from build123d import *

# Parameters (mm, degrees)
F3_DEPTH = 8
F4_R     = 0.4
F5_R     = 0.5


with BuildPart() as f1:
    # F0 (on Right) → F1 (revolve)
    with BuildSketch(Plane.YZ):
        Polygon((0, -60), (0, 0), (-7.95, 0), (-7.95, -10), (-5, -10), (-5, -60), align=None)
    revolve(axis=Axis((0, 0, -30), (0, 0, -1)))

    # F2 (on face) → F3 (cut)
    with BuildSketch(Plane.XY):
        Polygon((-2.341641, 3.981212), (-4.618651, -0.037314), (-2.277011, -4.018527), (2.341641, -3.981212), (4.618651, 0.037314), (2.277011, 4.018527), align=None)
    extrude(amount=-F3_DEPTH, mode=Mode.SUBTRACT)

    # F4
    f4_edges = [f1.edges().sort_by_distance(p)[0] for p in [
        (0, 7.95, 0),
        (0, 7.95, -10),
    ]]
    fillet(f4_edges, radius=F4_R)

    # F5
    f5_edges = [f1.edges().sort_by_distance(p)[0] for p in [
        (0, 5, -10),
        (0, 5, -60),
    ]]
    fillet(f5_edges, radius=F5_R)


solid = f1.part
Geometry: final body of the model. Coordinates: model frame, mm. A direction names the side the tool comes from. Coordinates: 2 decimals unless noted, no trailing zeros. Loops run counter-clockwise (first coordinate to the right, second up) from the corner with the lowest first, then second, coordinate; pieces in that order, holes last. Notation, with made-up numbers: (13.25, -29.5) - (28.25, -29.5) arc R6 ccw to (28.25, -25.5) - close; hole circle Ø6 at (-7.75, 74.5). An arc over 180 degrees is marked (long way). Put each result on its own line as item: value. Start each with the question number.
Q1. Pull-direction query (Y, two-part tool) for faces 1 (the flat face through (6, -1, -10)), 2 (the flat face through (3.464, 2, -3.944)), 3 (the cylindrical face through (7.76, 1.72, -5.06)); classes: released by +Y, released by -Y, zero draft, split by the parting line, or undercut.
Q2. Cut plane A-A, the plane x = 0. Return loops of the section in (y, z), and give its area (3 significant figures).
Q3. Pin query (flat end, axial travel): pin 1 Ø2 at (y, z) = (5.5, -7) entering from +X; pin 2 Ø6 at (x, y) = (6, -0.5) entering from +Z; pin 3 Ø3 at (y, z) = (2, -53.5) entering from +X; pin 4 Ø2.5 at (x, y) = (-1.5, -1) entering from +Z. Return the tip coordinate at first contact, or that it passes through.
Q4. Cut plane B-B, the plane z = -19. Return loops of the section in (x, y).
Q5. Line query: line 1 (X direction, y = 5.75, z = -5); line 2 (Z direction, x = 0, y = 0); line 3 (Y direction, x = 0.25, z = -2.5). Output: solid intervals per line, ascending.
Q6. Set-up query: faces 4 (the flat face through (-3.464, 2, -3.944)), 5 (the cylindrical face through (4.88, 1.08, -35.34)), 6 (the flat face through (0, 0, -60)). Return all of +Z, -Z, +X, -X, +Y, -Y with unobstructed straight access to the full face (end or side cutting, diameter ignored); none if empty.
Filled sheet:
1. face 1: zero draft
1. face 2: undercut
1. face 3: split by the parting line
2. outline: (-7.95, -9.6) arc R0.4 ccw to (-7.55, -10) - (-5.5, -10) arc R0.5 cw to (-5, -10.5) - (-5, -59.5) arc R0.5 ccw to (-4.5, -60) - (4.5, -60) arc R0.5 ccw to (5, -59.5) - (5, -10.5) arc R0.5 cw to (5.5, -10) - (7.55, -10) arc R0.4 ccw to (7.95, -9.6) - (7.95, -0.4) arc R0.4 ccw to (7.55, 0) - (4, 0) - (4, -8) - (-4, -8) - (-4, 0) - (-7.55, 0) arc R0.4 ccw to (-7.95, -0.4) - close
2. area: 595 mm²
3. pin 1: x = 6.55
3. pin 2: z = 0
3. pin 3: x = 4.97
3. pin 4: z = -8
4. outline: circle Ø10 at (0, 0)
5. line 1: -5.49 to 5.49
5. line 2: -60 to -8
5. line 3: -7.95 to -4, 4 to 7.95
6. face 4: +Z
6. face 5: -Z
6. face 6: -Z, +X, -X, +Y, -Y
